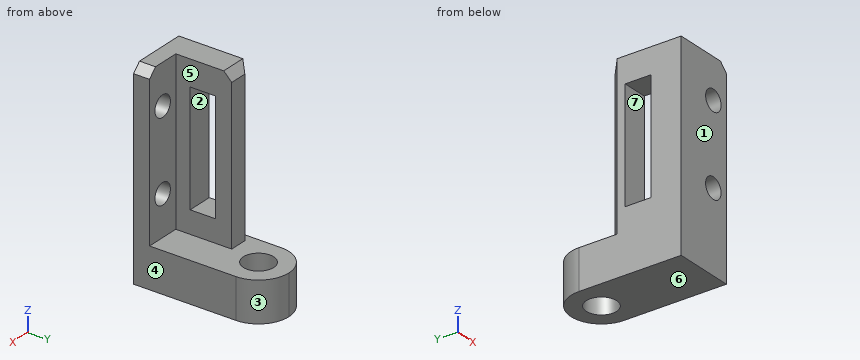
from build123d import *

# Parameters (mm, degrees)
BOSS_EXTRUDE1_DEPTH      = 19
BOSS_EXTRUDE1_DEPTH_BACK = 19
SKETCH2_W                = 16
SKETCH2_H                = 35
BOSS_EXTRUDE2_DEPTH      = 100
FILLET1_R                = 19
HOLE1_D                  = 19
CHAMFER1_SIZE            = 5
CHAMFER2_SIZE            = 5
SKETCH6_W                = 70
SKETCH6_H                = 16
CUT_EXTRUDE1_DEPTH       = 19
HOLE2_D                  = 13


with BuildPart() as part:
    # Sketch1 → Boss-Extrude1 (new, two sides: drawn at the far end of the back side and taken through both)
    with BuildSketch(Plane(origin=(0, 0, 0), x_dir=(0, 0, -1), z_dir=(1, 0, 0)).offset(-BOSS_EXTRUDE1_DEPTH_BACK)):
        Polygon((-62.5, 0), (62.5, 0), (62.5, 83), (37.5, 83), (37.5, 10), (-62.5, 10), align=None)
    extrude(amount=BOSS_EXTRUDE1_DEPTH + BOSS_EXTRUDE1_DEPTH_BACK)

    # Sketch2 → Boss-Extrude2 (add)
    with BuildSketch(Plane.XY.offset(-37.5)):
        with Locations((-11, 27.5)):
            Rectangle(SKETCH2_W, SKETCH2_H)
    extrude(amount=BOSS_EXTRUDE2_DEPTH)

    # Fillet1
    fillet1_edges = [part.edges().sort_by_distance(p)[0] for p in [
        (-19, 83, -50),
        (19, 83, -50),
    ]]
    fillet(fillet1_edges, radius=FILLET1_R - 0.0001)  # a hair under: the kernel refuses the full size

    # Hole1 (through all)
    with Locations(Plane.XY.offset(-37.5)):
        with Locations((0, 64)):
            Hole(HOLE1_D / 2)

    # Chamfer1
    chamfer1_edges = [part.edges().sort_by_distance(p)[0] for p in [
        (-19, 45, 12.5),
        (-11, 45, 62.5),
    ]]
    chamfer(chamfer1_edges, length=CHAMFER1_SIZE)

    # Chamfer2
    chamfer2_edges = [part.edges().sort_by_distance(p)[0] for p in [
        (19, 5, 62.5),
    ]]
    chamfer(chamfer2_edges, length=CHAMFER2_SIZE)

    # Sketch6 → Cut-Extrude1 (cut)
    with BuildSketch(Plane(origin=(-3, 0, 0), x_dir=(0, 0, -1), z_dir=(1, 0, 0))):
        with Locations((-11.5, 27)):
            Rectangle(SKETCH6_W, SKETCH6_H)
    extrude(amount=-CUT_EXTRUDE1_DEPTH, mode=Mode.SUBTRACT)

    # Hole2 (through all)
    with Locations(Plane(origin=(0, 10, 0), x_dir=(1, 0, 0), z_dir=(0, 1, 0))):
        with Locations((8, 12.5), (8, -37.5)):
            Hole(HOLE2_D / 2)


solid = part.part
Check sheet for the modelled part. Datum: model origin and axes. Units: mm. Face numbers are marked on the shaded views. A direction names the side the tool comes from. Give positions to 0.01 mm unless a question says otherwise; leave off trailing zeros. Loops run counter-clockwise (first coordinate to the right, second up) from the corner with the lowest first, then second, coordinate; pieces in that order, holes last. Notation, with made-up numbers: M 66,1.5 L 94,1.5 A14 ccw 94,21.5 Z; hole C -0.5,-33 d4. An arc over 180 degrees is marked long. Return JSON: item names as keys, results as strings. Group by question number.
1. Cross-section at A-A on z = 27. Record the boundary of the cut face in (x, y), plus the area to 4 significant figures.
2. Thickness scan on L1, parallel to Z at x = 8, y = 7.75; L2, parallel to Y at x = -5.5, z = 26.5; L3, parallel to Y at x = 0, z = -43.25. Record the ranges inside material, lowest first.
3. Mould release check, pull along Y, two halves, no side actions. Record for the marked faces 1, 2, 3 and 4: released by +Y, released by -Y, zero draft, split by the parting line, or undercut.
4. Cross-section at C-C on y = 8.5. Record the boundary of the cut face in (x, z), plus the area to 3 significant figures.
5. Tool access check on the marked faces 5, 6 and 7. Record the directions out of +Z, -Z, +X, -X, +Y, -Y that give a thin tool (end or side, any length) a straight path to the whole face; none if there is none.
6. Cross-section at D-D on x = 3. Record the boundary of the cut face in (y, z).
7. Go/stop test with flat-tipped pins: pin 1 (11 mm diameter, centred on x = 12.5, z = 27.5, fed in from +Y); pin 2 (8 mm diameter, centred on x = -13, z = 26, fed in from +Y); pin 3 (1.5 mm diameter, centred on x = 1, y = 14, fed in from +Z). Record where each tip stops, or that it passes through.
Return value:
{
 "1": {"outline": "M -19,0 L 19,0 L 19,10 L -3,10 L -3,19 L -19,19 Z; M -19,35 L -3,35 L -3,45 L -14,45 L -19,40 Z", "area": "671.5 mm^2"},
 "2": {"L1": "-62.5 to -19, -6 to 31, 44 to 62.5", "L2": "0 to 19, 35 to 45", "L3": "0 to 54.5, 73.5 to 83"},
 "3": {"face 1": "released by -Y", "face 2": "undercut", "face 3": "released by +Y", "face 4": "zero draft"},
 "4": {"outline": "M -19,-62.5 L 19,-62.5 L 19,57.5 L 14,62.5 L -19,62.5 Z; hole C 8,-12.5 d13; hole C 8,37.5 d13", "area": "4,470 mm^2"},
 "5": {"face 5": "+Z, +X, +Y", "face 6": "-Z, +X, -X, +Y, -Y", "face 7": "+X, -X"},
 "6": {"outline": "M 0,-62.5 L 54.99,-62.5 L 54.99,-37.5 L 10,-37.5 L 10,-16.65 L 0,-16.65 Z; M 0,-8.35 L 10,-8.35 L 10,33.35 L 0,33.35 Z; M 0,41.65 L 10,41.65 L 10,62.5 L 0,62.5 Z; M 73.01,-62.5 L 82.76,-62.5 L 82.76,-37.5 L 73.01,-37.5 Z"},
 "7": {"pin 1": "y = 10", "pin 2": "y = 45", "pin 3": "z = -37.5"}
}
